from build123d import *

# Parameters (mm, degrees)
RESSALTO_EXTRUS_O1_DEPTH = 6
ESBO_O2_W                = 6
ESBO_O2_H                = 6
CORTE_EXTRUS_O1_DEPTH    = 10


with BuildPart() as part:
    # Ressalto-extrus_o1: read off the stored shape, not the designer's step
    # Ressalto-extrus_o1 outline → Ressalto-extrus_o1 (new body)
    with BuildSketch(Plane.XY):
        Polygon((-3, 2.28086846), (-3, 5.552723944), (-7.778174593, 7.778174593), (-7.259013875, 3.006781996), (-11, 0), (-7.259060972, -3.006840593), (-7.778161938, -7.778187248), (-3.006781996, -7.259013875), (0, -11), (3.006781996, -7.259013875), (7.778174593, -7.778174593), (7.259013875, -3.006781996), (11, 0), (7.259013875, 3.006781996), (7.778174593, 7.778174593), (3, 5.552723944), (3, 2.28086846), align=None)
    extrude(amount=RESSALTO_EXTRUS_O1_DEPTH)

    # Esbo_o2 → Corte-extrus_o1 (cut)
    with BuildSketch(Plane.XY.offset(6)):
        with Locations((0, -0.71913154)):
            Rectangle(ESBO_O2_W, ESBO_O2_H)
    extrude(amount=-CORTE_EXTRUS_O1_DEPTH, mode=Mode.SUBTRACT)


solid = part.part
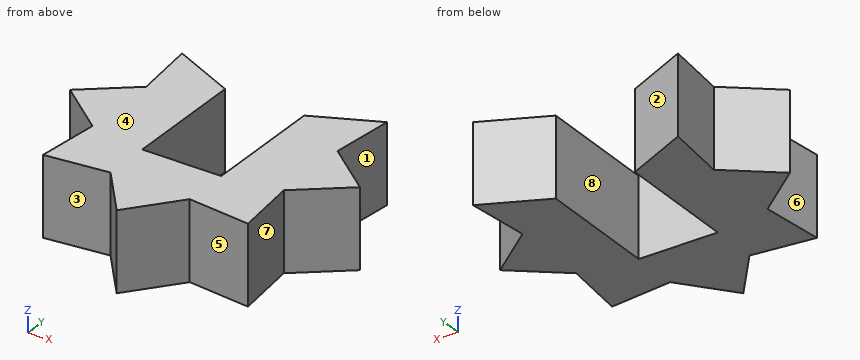
Work out the finished part from the listing and answer in its coordinate system (mm). Face numbers are marked on the shaded views. A direction names the side the tool comes from. Round coordinates to 2 decimals unless told otherwise and drop trailing zeros. Write each loop counter-clockwise with the first axis right and the second up, starting at its lowest first coordinate (ties: lowest second). Pieces come first, ordered by that corner, then holes. Notation, with made-up numbers: (89.25, -28) -> (94.25, -28) arc R35 cw to (94.25, 10) -> close; hole circle Ø9 at (78.25, 82). An arc over 180 degrees is marked (long way). Write each question's results on one line, items separated by ' | '.
Item 1: A flat-ended cylindrical pin translates along its axis: P1, Ø1.5, axis at x = 1, y = 4.5, coming from the -Z side. Find the tip coordinate at first contact, or state that the pin passes through.
Result set:
P1: through
Item 2: A cutting plane is placed at A-A, the plane z = 0.55. Determine the outline of the cut face in (x, y).
Result set:
outline: (-11, 0) -> (-7.26, -3.01) -> (-7.78, -7.78) -> (-3.01, -7.26) -> (0, -11) -> (3.01, -7.26) -> (7.78, -7.78) -> (7.26, -3.01) -> (11, 0) -> (7.26, 3.01) -> (7.78, 7.78) -> (3, 5.55) -> (3, -3.72) -> (-3, -3.72) -> (-3, 5.55) -> (-7.78, 7.78) -> (-7.26, 3.01) -> close
Item 3: A cutting plane is placed at D-D, the plane x = 9. Determine the outline of the cut face in (y, z).
Result set:
outline: (-1.61, 0) -> (1.61, 0) -> (1.61, 6) -> (-1.61, 6) -> close
Item 4: Which of the six approach directions +Z, -Z, +X, -X, +Y, -Y give full straight-line access (tool end or side, diameter ignored) to the marked faces 4, 5, 6, 7 and 8?
Result set:
face 4: +Z, +X, -X, +Y, -Y | face 5: +Z, -Z, -Y | face 6: +Z, -Z, -X | face 7: +Z, -Z, +X | face 8: +Z, -Z, +Y
Item 5: Find the intervals of material crossed by line 1 along X through (y, z) = (4.75, 2.5); line 2 along X through (y, z) = (-0.25, 0.8); line 3 along X through (y, z) = (-6.25, 5.6), in increasing order. Write a range as [from, to].
Result set:
line 1: [-7.45, -3], [3, 7.45] | line 2: [-10.69, -3], [3, 10.69] | line 3: [-7.61, 7.61]
Item 6: A cutting plane is placed at C-C, the plane y = 4.5. Determine the outline of the cut face in (x, z).
Result set:
outline: (-7.42, 0) -> (-3, 0) -> (-3, 6) -> (-7.42, 6) -> close; (3, 0) -> (7.42, 0) -> (7.42, 6) -> (3, 6) -> close
Item 7: A cutting plane is placed at B-B, the plane y = 0.25. Determine the outline of the cut face in (x, z).
Result set:
outline: (-10.69, 0) -> (-3, 0) -> (-3, 6) -> (-10.69, 6) -> close; (3, 0) -> (10.69, 0) -> (10.69, 6) -> (3, 6) -> close
Item 8: The mould has two halves that part along Y. Classify the marked faces 1, 2 and 3: +Y half, -Y half, draft (parallel to the pull), parting line (faces both ways), or undercut.
Result set:
face 1: undercut | face 2: +Y half | face 3: -Y half
